Read the model definition and answer for the solid it produces. Units are mm, in the model's axes. A direction names the side the tool comes from. Coordinates: 2 decimals unless noted, no trailing zeros. Write each loop counter-clockwise with the first axis right and the second up, starting at its lowest first coordinate (ties: lowest second). Pieces come first, ordered by that corner, then holes.
(1) Find the intervals of material crossed by probe 1 along Y at (x, z) = (-6.25, 105); probe 2 along Y at (x, z) = (-7, 246); probe 3 along Z at (x, y) = (-0.5, 6.5), in increasing order.
(2) Section C-C on y = 36.5 is taken. Write down the section's boundary in (x, z), then the cut area to 3 significant figures.
(3) Section A-A on z = 188.5 is taken. Write down the section's boundary in (x, y), then the cut area to 3 significant figures.
(4) The mould has two halves that part along Y. Classify faces 4 (the cylindrical face through (5.076, -9.759, 135.914)), 5 (the flat face through (0, 118, 322)), 6 (the cylindrical face through (-1.432, 128.906, 135.914)): +Y half, -Y half, draft (parallel to the pull), parting line (faces both ways), or undercut.
(5) Section D-D on z = 0 is taken. Write down the section's boundary in (x, y), then the cut area to 3 significant figures.
(6) Which of the six approach directions +Z, -Z, +X, -X, +Y, -Y give full straight-line access (tool end or side, diameter ignored) to faces 1 (the cylindrical face through (-2.38, 107.26, 303.27)), 2 (the cylindrical face through (2.38, 58.02, -10.74)), 3 (the flat face through (0, 0, 322))?
(7) Given pin 1 (5 mm diameter, centred on y = 5, z = 264.5, fed in from +X); pin 2 (1 mm diameter, centred on x = 8.5, z = 232.5, fed in from +Y); pin 3 (6 mm diameter, centred on x = -6, y = 42.5, fed in from -Z), each flat-ended and moving along its own axis, determine where each tip first touches the part or whether it passes through.
from build123d import *

# Parameters (mm, degrees)
SKETCH_1_R             = 11
EXTRUDE_1_DEPTH        = 287
SKETCH_2_R             = 11
EXTRUDE_2_DEPTH        = 118
PATTERN_LINEAR_1_COUNT = 2
PATTERN_LINEAR_1_PITCH = 118
CHAMFER_3_SIZE         = 21.999
SKETCH_3_R             = 10.9995
EXTRUDE_3_DEPTH        = 35
FILLET_1_R             = 2


with BuildPart() as part:
    # 草图1 → 拉伸1 (new body)
    with BuildSketch(Plane.XY):
        Circle(SKETCH_1_R)
    extrude_1 = extrude(amount=EXTRUDE_1_DEPTH)

    # 草图2 → 拉伸2 (add)
    with BuildSketch(Plane(origin=(0, 0, 0), x_dir=(1, 0, 0), z_dir=(0, 1, 0))):
        with Locations(Location((0, 0, 0), (0, 0, 180))):
            Circle(SKETCH_2_R)
    extrude(amount=EXTRUDE_2_DEPTH)

    # 阵列(线性)1: 拉伸1 ×2
    with Locations(*[(0, i * PATTERN_LINEAR_1_PITCH, 0) for i in range(1, PATTERN_LINEAR_1_COUNT)]):
        add(extrude_1)

    # 倒角3
    # the kernel refuses this chamfer: 21.999 mm, written as the material it adds along each edge
    with BuildSketch(Plane(origin=(67.574454052, 0, 0), x_dir=(0, -0.9996219169112966, 0.027495876610586372), z_dir=(-1, 0, 0))) as chamfer_3_piece_1_section:
        Polygon((CHAMFER_3_SIZE * 0.999621916911, -CHAMFER_3_SIZE * 0.0274958766106), (-CHAMFER_3_SIZE * 0.0274958766106, -CHAMFER_3_SIZE * 0.999621916911), (0, 0), align=None)
    chamfer_3_piece_1 = extrude(amount=135.148908105, mode=Mode.PRIVATE)
    chamfer_3_piece_1 = chamfer_3_piece_1 & Plane(origin=(0, 0, -4.859651136), x_dir=(1, 0, 0), z_dir=(0, 0, -1)) * Cylinder(11, 359, mode=Mode.PRIVATE)
    chamfer_3_piece_1 = chamfer_3_piece_1 & Plane(origin=(0, -4.859651136, 0), x_dir=(-1, 0, 0), z_dir=(0, -1, 0)) * Cylinder(11, 359, mode=Mode.PRIVATE)
    add(chamfer_3_piece_1)
    with BuildSketch(Plane(origin=(-67.574454052, 118, 0), x_dir=(0, -0.027495876610586358, -0.9996219169112966), z_dir=(1, 0, 0))) as chamfer_3_piece_2_section:
        Polygon((CHAMFER_3_SIZE * 0.999621916911, CHAMFER_3_SIZE * 0.0274958766106), (-CHAMFER_3_SIZE * 0.0274958766106, CHAMFER_3_SIZE * 0.999621916911), (0, 0), align=None)
    chamfer_3_piece_2 = extrude(amount=135.148908105, mode=Mode.PRIVATE)
    chamfer_3_piece_2 = chamfer_3_piece_2 & Plane(origin=(0, 122.859651136, 0), x_dir=(-1, 0, 0), z_dir=(0, -1, 0)) * Cylinder(11, 359, mode=Mode.PRIVATE)
    chamfer_3_piece_2 = chamfer_3_piece_2 & Plane(origin=(0, 118, -4.859651136), x_dir=(1, 0, 0), z_dir=(0, 0, -1)) * Cylinder(11, 359, mode=Mode.PRIVATE)
    add(chamfer_3_piece_2)

    # 草图3 → 拉伸3 (add)
    with BuildSketch(Plane.XY.offset(287)):
        with Locations((0, 118)):
            Circle(SKETCH_3_R)
        Circle(SKETCH_3_R)
    extrude(amount=EXTRUDE_3_DEPTH)

    # 圆角1
    fillet_1_edges = [part.edges().sort_by_distance(p)[0] for p in [
        (-10.9995, 118, 322),
        (-10.9995, 0, 322),
    ]]
    fillet(fillet_1_edges, radius=FILLET_1_R)


solid = part.part
Response:
1. probe 1: y = -9.05 to 9.05, 108.95 to 127.05
1. probe 2: y = -8.49 to 8.49, 109.51 to 126.49
1. probe 3: z = -10.99 to 322
2. outline: circle Ø22 at (0, 0)
2. area: 380 mm2
3. outline: circle Ø22 at (0, 0); circle Ø22 at (0, 118)
3. area: 760 mm2
4. face 4: undercut
4. face 5: draft
4. face 6: undercut
5. outline: (-11, 0) arc R11 ccw to (11, 0) - (11, 118) arc R11 ccw to (-11, 118) - close
5. area: 2,980 mm2
6. face 1: +Z
6. face 2: none
6. face 3: +Z, +X, -X, +Y, -Y
7. pin 1: stops at x = 10.71
7. pin 2: stops at y = 125.55
7. pin 3: stops at z = -10.58
